```python
from build123d import *

# Parameters (mm, degrees)
CROQUIS1_R              = 15
SALIENTE_EXTRUIR1_DEPTH = 27
CROQUIS2_R              = 11.5
SALIENTE_EXTRUIR2_DEPTH = 20
CHAFL_N1_SIZE           = 5
CHAFL_N1_SIZE2          = 2.331538291
CHAFL_N2_SIZE           = 5
CHAFL_N2_SIZE2          = 2.331538291
CROQUIS3_R              = 5
CORTAR_EXTRUIR1_DEPTH   = 10
CROQUIS4_R              = 3
CORTAR_EXTRUIR2_DEPTH   = 10


with BuildPart() as part:
    # Croquis1 → Saliente-Extruir1 (new body)
    with BuildSketch(Plane(origin=(0, 0, 0), x_dir=(1, 0, 0), z_dir=(0, 1, 0))):
        with Locations(Location((0, 0, 0), (0, 0, 270))):
            Circle(CROQUIS1_R)
    extrude(amount=SALIENTE_EXTRUIR1_DEPTH)

    # Croquis2 → Saliente-Extruir2 (add)
    with BuildSketch(Plane(origin=(0, 27, 0), x_dir=(1, 0, 0), z_dir=(0, 1, 0))):
        with Locations(Location((0, 0, 0), (0, 0, 270))):
            Circle(CROQUIS2_R)
    extrude(amount=SALIENTE_EXTRUIR2_DEPTH)

    # Chaflán1
    chafl_n1_edges = [part.edges().sort_by_distance(p)[0] for p in [
        (0, 47, -11.5),
    ]]
    chafl_n1_side = [part.faces().sort_by_distance(p)[0] for p in [
        (0, 37, -11.5),
    ]]
    chamfer(chafl_n1_edges, length=CHAFL_N1_SIZE, length2=CHAFL_N1_SIZE2, reference=chafl_n1_side[0])

    # Chaflán2
    chafl_n2_edges = [part.edges().sort_by_distance(p)[0] for p in [
        (0, 27, -15),
    ]]
    chafl_n2_side = [part.faces().sort_by_distance(p)[0] for p in [
        (0, 13.5, -15),
    ]]
    chamfer(chafl_n2_edges, length=CHAFL_N2_SIZE, length2=CHAFL_N2_SIZE2, reference=chafl_n2_side[0])

    # Croquis3 → Cortar-Extruir1 (cut)
    with BuildSketch(Plane(origin=(0, 0, 0), x_dir=(-1, 0, 0), z_dir=(0, -1, 0))):
        with Locations(Location((0, 0, 0), (0, 0, 90))):
            Circle(CROQUIS3_R)
    extrude(amount=-CORTAR_EXTRUIR1_DEPTH, mode=Mode.SUBTRACT)

    # Croquis4 → Cortar-Extruir2 (cut)
    with BuildSketch(Plane(origin=(0, 47, 0), x_dir=(1, 0, 0), z_dir=(0, 1, 0))):
        with Locations(Location((0, 0, 0), (0, 0, 270))):
            Circle(CROQUIS4_R)
    extrude(amount=-CORTAR_EXTRUIR2_DEPTH, mode=Mode.SUBTRACT)


solid = part.part
```
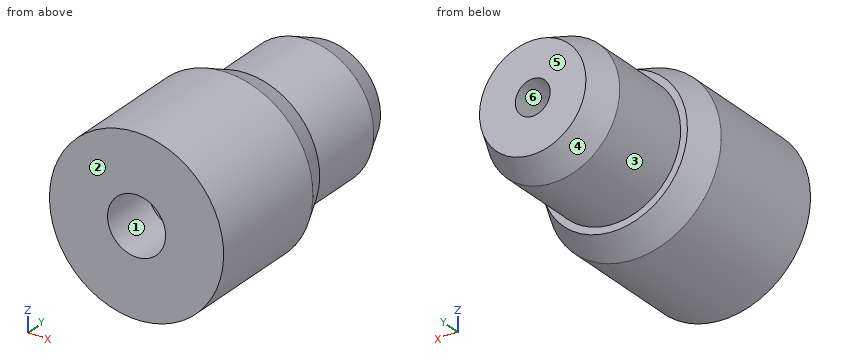
Read the model definition and answer for the solid it produces. Units are mm, in the model's axes. Face numbers are marked on the shaded views. A direction names the side the tool comes from. Round coordinates to 2 decimals unless told otherwise and drop trailing zeros. Write each loop counter-clockwise with the first axis right and the second up, starting at its lowest first coordinate (ties: lowest second). Pieces come first, ordered by that corner, then holes. Notation, with made-up numbers: (-34.75, 74.5) - (-23.75, 74.5) arc R13 cw to (-23.75, 84.5) - close; hole circle Ø7 at (-33.5, 21.25). An arc over 180 degrees is marked (long way). Use CSV: the item, a comma, the result in double quotes.
Q1. Find section A-A, the plane x = 0. Write down the section's boundary in (y, z), then the cut area to 3 significant figures.
Values:
outline,"(0, -15) - (22, -15) - (27, -12.67) - (27, -11.5) - (42, -11.5) - (47, -9.17) - (47, -3) - (37, -3) - (37, 3) - (47, 3) - (47, 9.17) - (42, 11.5) - (27, 11.5) - (27, 12.67) - (22, 15) - (0, 15) - (0, 5) - (10, 5) - (10, -5) - (0, -5) - close"
area,"1,090 mm²"
Q2. Each of these flat-tipped pins is pushed along its axis until it touches: pin 1 Ø2 at (y, z) = (38.5, -2) entering from +X; pin 2 Ø5 at (x, y) = (4.5, 38.5) entering from +Z; pin 3 Ø5 at (x, z) = (0, 0) entering from +Y. Where does it stop, or does it pass through?
Values:
pin 1,"stops at x = 11.46"
pin 2,"stops at z = 11.32"
pin 3,"stops at y = 37"
Q3. A tool of negligible diameter and unlimited length cuts with its end or side. For the marked faces 1, 2 and 3, from which of +Z, -Z, +X, -X, +Y, -Y can it reach the whole face along a straight path? Write none if from no direction.
Values:
face 1,"-Y"
face 2,"+Z, -Z, +X, -X, -Y"
face 3,"+Y"
Q4. Find section B-B, the plane z = 0. Write down the section's boundary in (x, y), then the cut area to 3 significant figures.
Values:
outline,"(-15, 0) - (-5, 0) - (-5, 10) - (5, 10) - (5, 0) - (15, 0) - (15, 22) - (12.67, 27) - (11.5, 27) - (11.5, 42) - (9.17, 47) - (3, 47) - (3, 37) - (-3, 37) - (-3, 47) - (-9.17, 47) - (-11.5, 42) - (-11.5, 27) - (-12.67, 27) - (-15, 22) - close"
area,"1,090 mm²"
Q5. Straight lines are drawn through the part: line 1 along Y through (x, z) = (-8.75, 8.5); line 2 along X through (y, z) = (4.25, 0); line 3 along X through (y, z) = (42.25, 0). For each, find the intervals that lie inside material, in ascending order.
Values:
line 1,"y = 0 to 27"
line 2,"x = -15 to -5, 5 to 15"
line 3,"x = -11.38 to -3, 3 to 11.38"
Q6. Find section D-D, the plane y = 31. Write down the section's boundary in (x, z), then the cut area to 3 significant figures.
Values:
outline,"circle Ø23 at (0, 0)"
area,"415 mm²"
Q7. Determine the mould class of the marked faces 4, 5 and 6 for opening direction Z: +Z half, -Z half, draft (parallel to the pull), parting line (faces both ways), or undercut.
Values:
face 4,"parting line"
face 5,"draft"
face 6,"undercut"
Q8. Find section C-C, the plane y = 9. Write down the section's boundary in (x, z).
Values:
outline,"circle Ø30 at (0, 0); hole circle Ø10 at (0, 0)"
